Source: three-view drawing plus pictorial views. Frame: mm from the lowest corner of the part. Coordinates: 2 decimals unless noted, no trailing zeros. Write each loop counter-clockwise with the first axis right and the second up, starting at its lowest first coordinate (ties: lowest second). Pieces come first, ordered by that corner, then holes. Notation, with made-up numbers: (57.5, 65) - (84.5, 65) arc R37 ccw to (84.5, 102) - close; hole circle Ø9 at (63.25, 79.5). An arc over 180 degrees is marked (long way). Put each result on its own line as item: value.
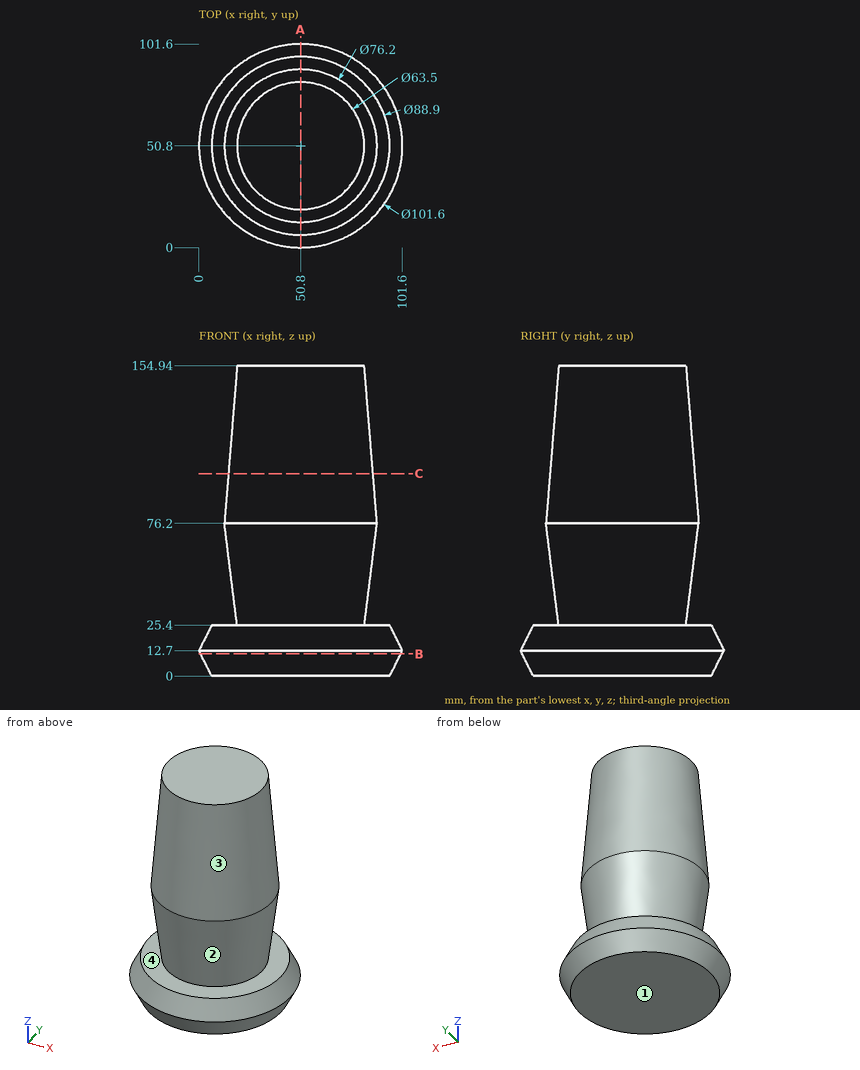
1. Pin query (flat end, axial travel): pin 1 Ø5 at (x, y) = (83.5, 59) entering from +Z; pin 2 Ø2 at (y, z) = (77.5, 123) entering from -X; pin 3 Ø1 at (x, z) = (39.5, 122.5) entering from +Y; pin 4 Ø4 at (x, z) = (84, 129) entering from -Y. Return the tip coordinate at first contact, or that it passes through.
Answer below:
pin 1: stops at z = 154.94
pin 2: stops at x = 28.04
pin 3: stops at y = 83.43
pin 4: stops at y = 37.67
2. Section query A-A (x = 50.8). Return loops of the section in (y, z), then the cut area to 3 significant figures.
Answer below:
outline: (0, 12.7) - (6.35, 0) - (95.25, 0) - (101.6, 12.7) - (95.25, 25.4) - (82.55, 25.4) - (88.9, 76.2) - (82.55, 154.94) - (19.05, 154.94) - (12.7, 76.2) - (19.05, 25.4) - (6.35, 25.4) - close
area: 11,500 mm²
3. Section query C-C (z = 101). Return loops of the section in (x, y).
Answer below:
outline: circle Ø72.2 at (50.8, 50.8)
4. Ray query, probe 1 along Z at (x, y) = (91, 38); probe 2 along Y at (x, z) = (24, 122); probe 3 along Y at (x, z) = (18, 84). Return the intervals inside material, ascending. Write a range as from..to.
Answer below:
probe 1: z = 0..25.4
probe 2: y = 29.22..72.38
probe 3: y = 32.68..68.92
5. Mould query, pull axis Z, two halves, no side actions, for the marked faces 1, 2, 3 and 4. Classes: +Z half, -Z half, draft (parallel to the pull), parting line (faces both ways), or undercut.
Answer below:
face 1: -Z half
face 2: undercut
face 3: +Z half
face 4: undercut
6. Section query B-B (z = 11). Return loops of the section in (x, y).
Answer below:
outline: circle Ø99.9 at (50.8, 50.8)
